Check sheet for the drawn part. Datum: minimum x, y, z corner. Units: mm. Coordinates: 2 decimals unless noted, no trailing zeros. Write each loop counter-clockwise with the first axis right and the second up, starting at its lowest first coordinate (ties: lowest second). Pieces come first, ordered by that corner, then holes. Notation, with made-up numbers: M -35.75,-18 L 14.25,-18 A33 cw 14.25,16 Z; hole C 88,75.25 d1. An arc over 180 degrees is marked long. Write item = value, one per line. Start each with the question number.
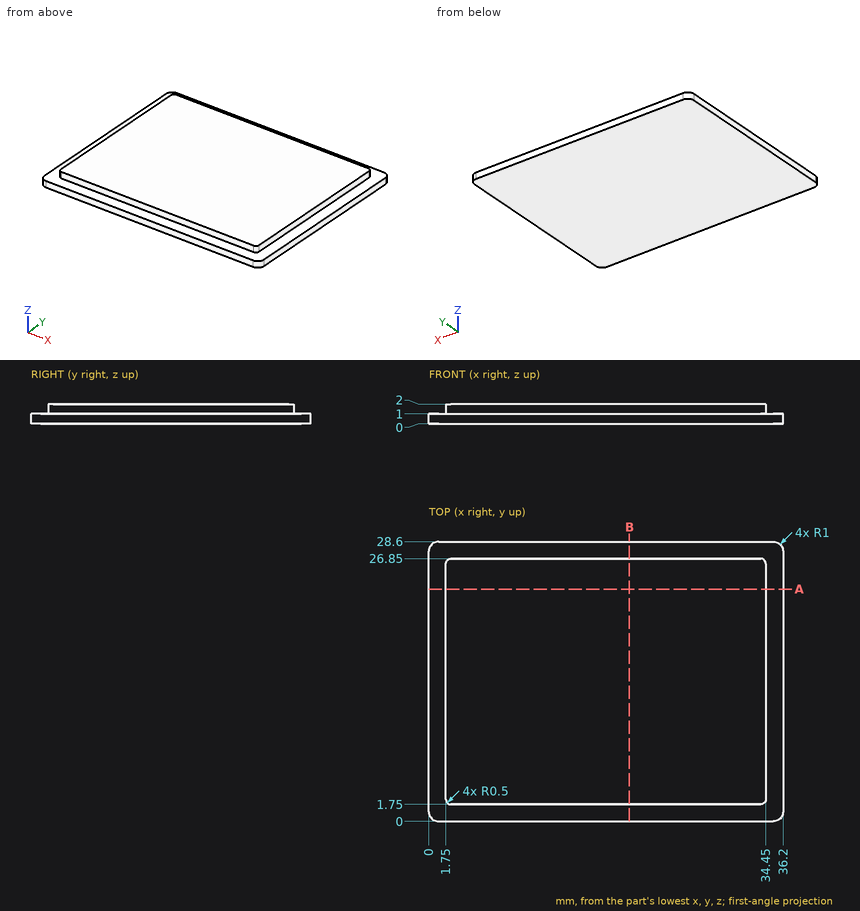
Q1. Cross-section at B-B on x = 20.5. Enter the section's corners in (y, z), and give its area (3 significant figures).
Q2. Scan lines: L1, parallel to X at y = 14, z = 1.75; L2, parallel to Y at x = 13, z = 1.55; L3, parallel to Z at x = 7.5, y = 27.25. Record each from-to range of solid material in increasing order.
Q3. Cross-section at A-A on y = 23.75. Enter the section's corners in (x, z).
Q4. Gauge pin test, flat ends, axial feed: pin 1 (0.8 mm diameter, centred on x = 14.5, z = 1.5, fed in from -Y); pin 2 (0.5 mm diameter, centred on y = 18, z = 1.5, fed in from -X). Record the tip position at first contact, or that the pin passes through.
Values found:
q1.outline = M 0,0 L 28.6,0 L 28.6,1 L 26.85,1 L 26.85,2 L 1.75,2 L 1.75,1 L 0,1 Z
q1.area = 53.7 mm²
q2.L1 = 1.75 to 34.45
q2.L2 = 1.75 to 26.85
q2.L3 = 0 to 1
q3.outline = M 0,0 L 36.2,0 L 36.2,1 L 34.45,1 L 34.45,2 L 1.75,2 L 1.75,1 L 0,1 Z
q4.pin_1 = 1.75
q4.pin_2 = 1.75
